Geometry check sheet. Reference: the model listing, model coordinates, mm. Face numbers are marked on the shaded views. A direction names the side the tool comes from. Round coordinates to 2 decimals unless told otherwise and drop trailing zeros. Write each loop counter-clockwise with the first axis right and the second up, starting at its lowest first coordinate (ties: lowest second). Pieces come first, ordered by that corner, then holes.
Item 1: Cross-section at A-A (y = 0). Enter the section's corners in (x, z).
Item 2: Access from +Z, -Z, +X, -X, +Y, -Y to the whole of each face (thin tool, end or side, straight path). Record for the marked faces 1, 2 and 3.
Item 3: Cross-section at B-B (x = -10). Enter the section's corners in (y, z).
Item 4: Scan lines: probe 1 along Y at (x, z) = (2.25, 0); probe 2 along Z at (x, y) = (1.2, 24); probe 3 along Y at (x, z) = (0, 0.35). Record each from-to range of solid material in increasing order.
Item 5: Cross-section at C-C (y = 24). Enter the section's corners in (x, z), then the cut area to 3 significant figures.
Item 6: Cross-section at D-D (z = 0.5). Enter the section's corners in (x, y), then the cut area to 3 significant figures.
Item 7: Depth check by flat-ended pin: P1, Ø7, axis at x = -36, z = -7, coming from the +Y side; P2, Ø5, axis at y = 24, z = 0, coming from the +X side; P3, Ø1.5, axis at x = -28, z = 0, coming from the -Y side. Enter the tip coordinate at first touch or a pass-through.
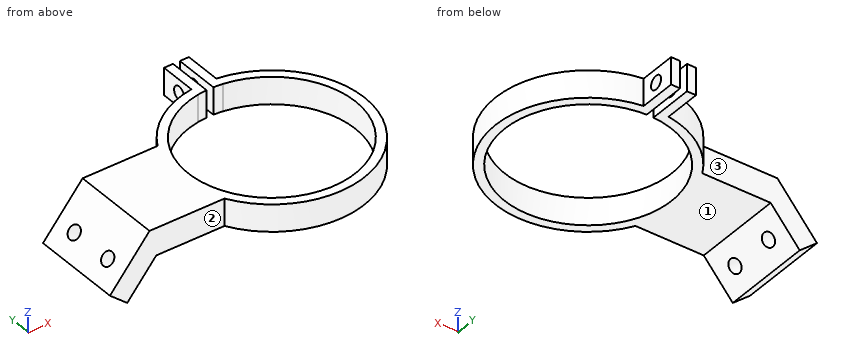
from build123d import *

# Parameters (mm, degrees)
BOSS_EXTRUDE1_DEPTH             = 3
SKETCH2_R                       = 1.5
CUT_EXTRUDE1_DEPTH              = 21.5
CUT_EXTRUDE1_DEPTH_BACK         = 35.5
BOSS_EXTRUDE2_REACH             = 30.5
BOSS_EXTRUDE2_DIRECTION_2_REACH = 22.5
SKETCH4_R                       = 1.5
CUT_EXTRUDE2_DEPTH              = 46.913208795
CUT_EXTRUDE2_DEPTH_BACK         = 12.714884867


with BuildPart() as part:
    # Sketch1 → Boss-Extrude1 (new body, symmetric)
    with BuildSketch(Plane.XY):
        with BuildLine():
            ThreePointArc((20.5, 0), (15.437373481, 13.48842096), (2.75, 20.314711418))
            Line((2.75, 20.314711418), (2.75, 18.294466376))
            ThreePointArc((2.75, 18.294466376), (14.020074893, 12.070107705), (18.5, 0))
            ThreePointArc((18.5, 0), (-12.070107705, -14.020074893), (-2.75, 18.294466376))
            Line((-2.75, 18.294466376), (-2.75, 20.314711418))
            ThreePointArc((-2.75, 20.314711418), (-11.53940193, 16.943795416), (-17.895530168, 10))
            ThreePointArc((-17.895530168, 10), (-20.5, 0), (-17.895530168, -10))
            ThreePointArc((-17.895530168, -10), (5.166799374, -19.838200126), (20.5, 0))
        make_face()
        with BuildLine():
            ThreePointArc((2.75, 20.314711418), (1.752101194, 20.424988162), (0.75, 20.486275894))
            Line((0.75, 20.486275894), (0.75, 18.484791046))
            ThreePointArc((0.75, 18.484791046), (1.752585481, 18.416797879), (2.75, 18.294466376))
            Line((2.75, 18.294466376), (2.75, 20.314711418))
        make_face()
        with BuildLine():
            Line((-0.75, 18.484791046), (-0.75, 20.486275894))
            ThreePointArc((-0.75, 20.486275894), (-1.752101194, 20.424988162), (-2.75, 20.314711418))
            Line((-2.75, 20.314711418), (-2.75, 18.294466376))
            ThreePointArc((-2.75, 18.294466376), (-1.752585481, 18.416797879), (-0.75, 18.484791046))
        make_face()
        with BuildLine():
            ThreePointArc((-2.75, 20.314711418), (-1.752101194, 20.424988162), (-0.75, 20.486275894))
            Line((-0.75, 20.486275894), (-0.75, 28.5))
            Line((-0.75, 28.5), (-2.75, 28.5))
            Line((-2.75, 28.5), (-2.75, 25.5))
            Line((-2.75, 25.5), (-2.75, 22.5))
            Line((-2.75, 22.5), (-2.75, 20.314711418))
        make_face()
        with BuildLine():
            Line((2.75, 25.5), (2.75, 28.5))
            Line((2.75, 28.5), (0.75, 28.5))
            Line((0.75, 28.5), (0.75, 20.486275894))
            ThreePointArc((0.75, 20.486275894), (1.752101194, 20.424988162), (2.75, 20.314711418))
            Line((2.75, 20.314711418), (2.75, 22.5))
            Line((2.75, 22.5), (2.75, 25.5))
        make_face()
        with BuildLine():
            Line((-20.5, -10), (-17.895530168, -10))
            ThreePointArc((-17.895530168, -10), (-20.5, 0), (-17.895530168, 10))
            Line((-17.895530168, 10), (-20.5, 10))
            Line((-20.5, 10), (-34.5, 10))
            Line((-34.5, 10), (-34.5, -10))
            Line((-34.5, -10), (-20.5, -10))
        make_face()
    extrude(amount=BOSS_EXTRUDE1_DEPTH, both=True)

    # Sketch2 → Cut-Extrude1 (cut, two sides)
    with BuildSketch(Plane(origin=(0, 0, 0), x_dir=(0, 0, -1), z_dir=(1, 0, 0))) as cut_extrude1_sk:
        with Locations((0, 24)):
            Circle(SKETCH2_R)
    extrude(amount=CUT_EXTRUDE1_DEPTH, mode=Mode.SUBTRACT)
    extrude(cut_extrude1_sk.sketch, amount=-CUT_EXTRUDE1_DEPTH_BACK, mode=Mode.SUBTRACT)

    # Boss-Extrude2: up to this face of the body (flat: up to its plane)
    boss_extrude2_end = Plane(part.part.faces().sort_by_distance((-26.197765084, 10, 0))[0])
    # Sketch3 → Boss-Extrude2 (add, up to the picked face)
    with BuildSketch(Plane(origin=(0, 0, 0), x_dir=(1, 0, 0), z_dir=(0, 1, 0)), mode=Mode.PRIVATE) as boss_extrude2_sk1:
        Polygon((-34.5, -3), (-43.265659653, 7.446506383), (-39.435437437, 10.660444431), (-33.00756134, 3), align=None)
    boss_extrude2_tool1 = split(extrude(boss_extrude2_sk1.sketch, amount=BOSS_EXTRUDE2_REACH, mode=Mode.PRIVATE), bisect_by=boss_extrude2_end, keep=Keep.BOTH, mode=Mode.PRIVATE)
    add(boss_extrude2_tool1.solids().sort_by_distance((-37.620413, 0, -4.408594))[0])

    # Boss-Extrude2 direction 2: up to this face of the body (flat: up to its plane)
    boss_extrude2_direction_2_end = Plane(part.part.faces().sort_by_distance((-26.197765084, -10, 0))[0])
    # Sketch3 → Boss-Extrude2 direction 2 (add, up to the picked face)
    with BuildSketch(Plane(origin=(0, 0, 0), x_dir=(1, 0, 0), z_dir=(0, 1, 0)), mode=Mode.PRIVATE) as boss_extrude2_direction_2_sk1:
        Polygon((-34.5, -3), (-43.265659653, 7.446506383), (-39.435437437, 10.660444431), (-33.00756134, 3), align=None)
    boss_extrude2_direction_2_tool1 = split(extrude(boss_extrude2_direction_2_sk1.sketch, amount=-BOSS_EXTRUDE2_DIRECTION_2_REACH, mode=Mode.PRIVATE), bisect_by=boss_extrude2_direction_2_end, keep=Keep.BOTH, mode=Mode.PRIVATE)
    add(boss_extrude2_direction_2_tool1.solids().sort_by_distance((-37.620413, 0, -4.408594))[0])

    # Sketch4 → Cut-Extrude2 (cut, two sides)
    with BuildSketch(Plane(origin=(-17.892420479, 0, 15.013523425), x_dir=(-0.64278761, 0, -0.766044443), z_dir=(0.766044443, 0, -0.64278761))) as cut_extrude2_sk:
        with Locations((28.514984785, 5)):
            Circle(SKETCH4_R)
        with Locations((28.514984785, -5)):
            Circle(SKETCH4_R)
    extrude(amount=CUT_EXTRUDE2_DEPTH, mode=Mode.SUBTRACT)
    extrude(cut_extrude2_sk.sketch, amount=-CUT_EXTRUDE2_DEPTH_BACK, mode=Mode.SUBTRACT)


solid = part.part
Resolved:
1. outline: (-43.27, -7.45) - (-39.44, -10.66) - (-33.01, -3) - (-18.5, -3) - (-18.5, 3) - (-34.5, 3) - close; (18.5, -3) - (20.5, -3) - (20.5, 3) - (18.5, 3) - close
2. face 1: -Z, +X, +Y, -Y
2. face 2: +Z, -Z, -X, -Y
2. face 3: +Z, -Z, -X, +Y
3. outline: (-17.9, -3) - (-15.56, -3) - (-15.56, 3) - (-17.9, 3) - close; (15.56, -3) - (17.9, -3) - (17.9, 3) - (15.56, 3) - close
4. probe 1: y = -20.38 to -18.36, 18.36 to 22.5, 25.5 to 28.5
4. probe 2: z = -3 to -1.5, 1.5 to 3
4. probe 3: y = -20.5 to -18.5
5. outline: (-2.75, -3) - (-0.75, -3) - (-0.75, -1.5) - (-2.75, -1.5) - close; (-2.75, 1.5) - (-0.75, 1.5) - (-0.75, 3) - (-2.75, 3) - close; (0.75, -3) - (2.75, -3) - (2.75, -1.5) - (0.75, -1.5) - close; (0.75, 1.5) - (2.75, 1.5) - (2.75, 3) - (0.75, 3) - close
5. area: 12.0 mm2
6. outline: (-36.6, -10) - (-17.9, -10) arc R20.5 ccw (long way) to (2.75, 20.31) - (2.75, 22.59) - (0.75, 22.59) - (0.75, 18.48) arc R18.5 cw (long way) to (-0.75, 18.48) - (-0.75, 22.59) - (-2.75, 22.59) - (-2.75, 20.31) arc R20.5 ccw to (-17.9, 10) - (-36.6, 10) - close; (-2.75, 25.41) - (-0.75, 25.41) - (-0.75, 28.5) - (-2.75, 28.5) - close; (0.75, 25.41) - (2.75, 25.41) - (2.75, 28.5) - (0.75, 28.5) - close
6. area: 602 mm2
7. P1: stops at y = 10
7. P2: stops at x = 2.75
7. P3: stops at y = -10
